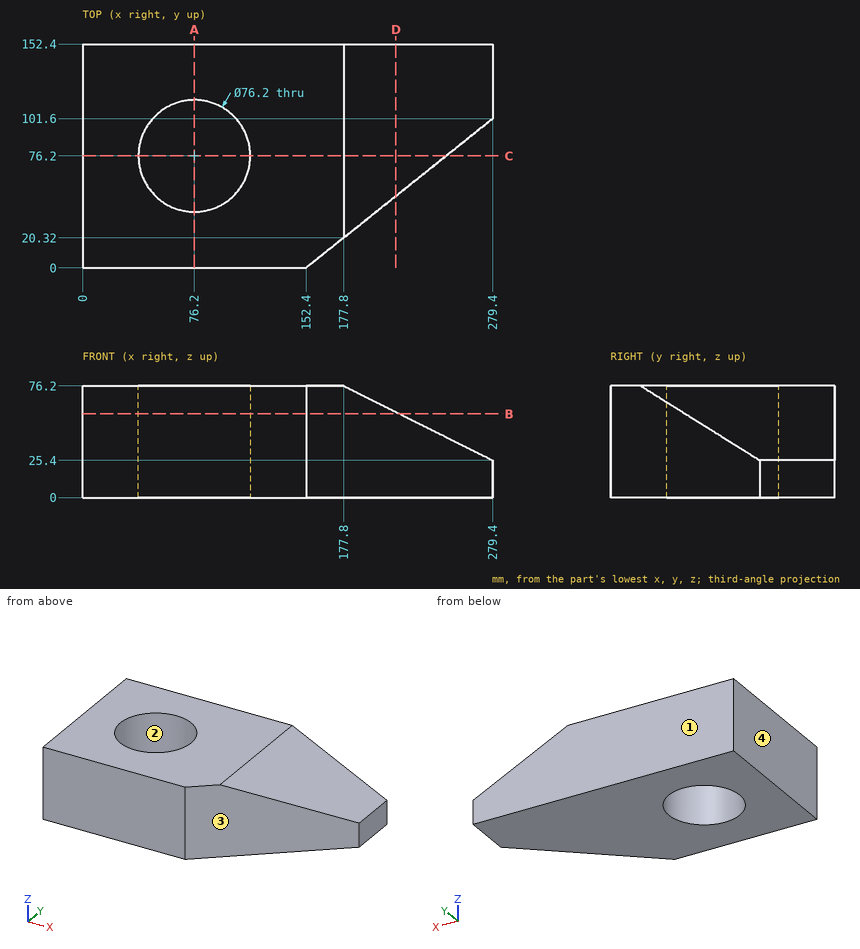
Drawing for the job (mm, zero at the part's lowest x, y, z). Give positions to 0.01 mm unless a question says otherwise; leave off trailing zeros. Order: outer loops, then holes, each group sorted by start corner. A loop starts at its lowest first (then second) coordinate and runs counter-clockwise, first axis right, second up. Notation, with made-up numbers: M 65,69.5 L 91,69.5 A23 ccw 91,98.5 Z; hole C -4.75,22 d10. An arc over 180 degrees is marked long. Use a Markdown table: item, result. Add a question column.
(1) Saw through at A-A, the plane x = 76.2. Give the cut face in (y, z).
(2) Saw through at D-D, the plane x = 213.5. Give the cut face in (y, z).
(3) Mould opens along X. For the marked faces 1, 2, 3 and 4 say: +X half, -X half, draft (parallel to the pull), parting line (faces both ways), or undercut.
(4) Saw through at B-B, the plane z = 57. Give the cut face in (x, y).
(5) Saw through at C-C, the plane y = 76.2. Give the cut face in (x, z) (3 decimals), and give its area (3 significant figures).
(6) Drop flat-ended pins along their axis: P1, Ø12, axis at y = 89.5, z = 55.5, coming from the +X side; P2, Ø1, axis at y = 86.5, z = 37.5, coming from the +X side; P3, Ø3, axis at y = 60, z = 12.5, coming from the +X side (3 decimals). Give the stop position or say it passes through.
(7) Probe line 1 along Y through (x, z) = (76.2, 20); line 2 along X through (y, z) = (76, 41); line 3 along X through (y, z) = (60.5, 37.5) (3 decimals). List the from-to ranges inside material, lowest first. Write a range as [from, to].
Answer key:
| question | item | result |
|---|---|---|
| 1 | outline | M 0,0 L 38.1,0 L 38.1,76.2 L 0,76.2 Z; M 114.3,0 L 152.4,0 L 152.4,76.2 L 114.3,76.2 Z |
| 2 | outline | M 48.88,0 L 152.4,0 L 152.4,58.35 L 48.88,58.35 Z |
| 3 | face 1 | draft |
| 3 | face 2 | undercut |
| 3 | face 3 | +X half |
| 3 | face 4 | -X half |
| 4 | outline | M 0,0 L 152.4,0 L 216.2,51.04 L 216.2,152.4 L 0,152.4 Z; hole C 76.2,76.2 d76.2 |
| 5 | outline | M 0,0 L 38.1,0 L 38.1,76.2 L 0,76.2 Z; M 114.3,0 L 247.65,0 L 247.65,41.275 L 177.8,76.2 L 114.3,76.2 Z |
| 5 | area | 11,800 mm^2 |
| 6 | P1 | x = 231.2 |
| 6 | P2 | x = 256.2 |
| 6 | P3 | x = 229.275 |
| 7 | line 1 | [0, 38.1], [114.3, 152.4] |
| 7 | line 2 | [0, 38.1], [114.3, 247.4] |
| 7 | line 3 | [0, 41.485], [110.915, 228.025] |
